For this review, take the finished solid that the model builds, in its own axes (mm). Round coordinates to 2 decimals unless told otherwise and drop trailing zeros. Loops run counter-clockwise (first coordinate to the right, second up) from the corner with the lowest first, then second, coordinate; pieces in that order, holes last.
1) Wall thickness on L1, parallel to X at y = 441.5, z = -268.5; L2, parallel to Z at x = 373, y = 426.5; L3, parallel to Y at x = 908, z = -564.5: over which ranges is each line inside the solid? List them lowest first.
2) Insertion check: pin 1 (1.5 mm diameter, centred on x = 175.5, y = 107, fed in from -Z). The pin has a flat end and moves straight along its axis. Give the tip position at first contact, or say it passes through.
3) Take a section at C-C (x = -2). State the section outline as (y, z) points.
4) Take a section at A-A (y = -364). State the section outline as (x, z) points, then the cut area to 3 significant figures.
5) Take a section at B-B (z = -565). State the section outline as (x, y) points.
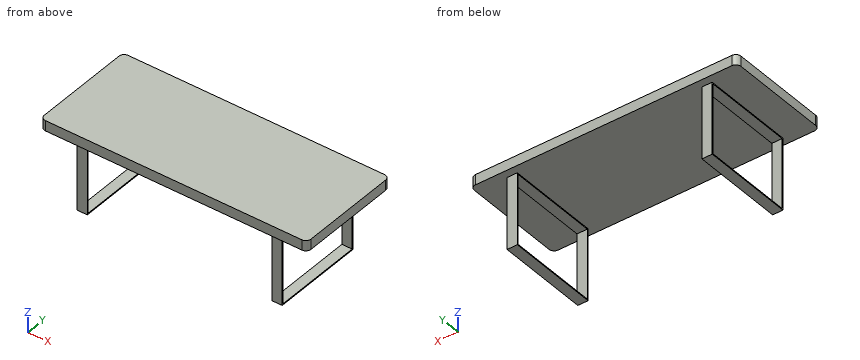
```python
from build123d import *

# Parameters (mm, degrees)
F0_W          = 2600
F0_H          = 1050
F1_DEPTH      = 100
F2_W          = 900
F2_H          = 700
F2_W_2        = 880
F2_H_2        = 680
F3_DEPTH      = 1000
F4_W          = 1800
F4_H          = 700
F5_DEPTH      = 525.001
F5_DEPTH_BACK = 525.001
F6_R          = 50


with BuildPart() as f1:
    # F0 (on Top) → F1 (new body)
    with BuildSketch(Plane.XY):
        Rectangle(F0_W, F0_H)
    extrude(amount=F1_DEPTH)

    # F2 (on Right) → F3 (join, symmetric)
    with BuildSketch(Plane.YZ):
        with Locations((0, -350)):
            Rectangle(F2_W, F2_H)
        with Locations((0, -350)):
            Rectangle(F2_W_2, F2_H_2, mode=Mode.SUBTRACT)
    extrude(amount=F3_DEPTH, both=True)

    # F4 (on Front) → F5 (cut, two sides)
    with BuildSketch(Plane.XZ) as f5_sk:
        with Locations((0, -350)):
            Rectangle(F4_W, F4_H)
    extrude(amount=-F5_DEPTH, mode=Mode.SUBTRACT)
    extrude(f5_sk.sketch, amount=F5_DEPTH_BACK, mode=Mode.SUBTRACT)

    # F6
    f6_edges = [f1.edges().sort_by_distance(p)[0] for p in [
        (1300, -525, 50),
        (1300, 525, 50),
        (-1300, 525, 50),
        (-1300, -525, 50),
    ]]
    fillet(f6_edges, radius=F6_R)


solid = f1.part
```
Response:
1. L1: x = -1000 to -900, 900 to 1000
1. L2: z = 0 to 100
1. L3: y = -450 to -440, 440 to 450
2. pin 1: stops at z = 0
3. outline: (-525, 0) - (525, 0) - (525, 100) - (-525, 100) - close
4. outline: (-1300, 0) - (-1000, 0) - (-1000, -10) - (-900, -10) - (-900, 0) - (900, 0) - (900, -10) - (1000, -10) - (1000, 0) - (1300, 0) - (1300, 100) - (-1300, 100) - close; (-1000, -700) - (-900, -700) - (-900, -690) - (-1000, -690) - close; (900, -700) - (1000, -700) - (1000, -690) - (900, -690) - close
4. area: 264,000 mm2
5. outline: (-1000, -450) - (-900, -450) - (-900, -440) - (-1000, -440) - close; (-1000, 440) - (-900, 440) - (-900, 450) - (-1000, 450) - close; (900, -450) - (1000, -450) - (1000, -440) - (900, -440) - close; (900, 440) - (1000, 440) - (1000, 450) - (900, 450) - close
